```python
from build123d import *

# Parameters (mm, degrees)
CROQUIS1_R                   = 5.9
SALIENTE_EXTRUIR1_DEPTH      = 32.5
CORTAR_EXTRUIR1_DEPTH        = 24
CORTAR_EXTRUIR_L_MINA1_START = -6.5
CROQUIS3_R                   = 5.8
CROQUIS3_R_2                 = 5
CORTAR_EXTRUIR_L_MINA1_DEPTH = 3
CROQUIS4_W                   = 7
CROQUIS4_H                   = 7
SALIENTE_EXTRUIR2_DEPTH      = 7
CROQUIS6_R                   = 1.75
CORTAR_EXTRUIR3_DEPTH        = 10.4
CORTAR_EXTRUIR4_DEPTH        = 18


with BuildPart() as part:
    # Croquis1 → Saliente-Extruir1 (new body, symmetric)
    with BuildSketch(Plane.XY):
        Circle(CROQUIS1_R)
    extrude(amount=SALIENTE_EXTRUIR1_DEPTH, both=True)

    # Croquis2 → Cortar-Extruir1 (cut)
    with BuildSketch(Plane.XY):
        with BuildLine():
            Line((-5.9, 0), (5.9, 0))
            ThreePointArc((5.9, 0), (0, 5.9), (-5.9, 0))
        make_face()
    extrude(amount=-CORTAR_EXTRUIR1_DEPTH, mode=Mode.SUBTRACT)

    # Croquis3 → Cortar-Extruir-L_mina1 (cut)
    with BuildSketch(Plane.XY.offset(32.5).offset(CORTAR_EXTRUIR_L_MINA1_START)):
        Circle(CROQUIS3_R)
        Circle(CROQUIS3_R_2, mode=Mode.SUBTRACT)
    extrude(amount=-CORTAR_EXTRUIR_L_MINA1_DEPTH, mode=Mode.SUBTRACT)

    # Croquis4 → Saliente-Extruir2 (add)
    with BuildSketch(Plane.XY.offset(32.5)):
        Rectangle(CROQUIS4_W, CROQUIS4_H)
    extrude(amount=SALIENTE_EXTRUIR2_DEPTH)

    # Croquis6 → Cortar-Extruir3 (cut, through all)
    with BuildSketch(Plane.ZY.offset(3.5)):
        with Locations((36.5, 0)):
            Circle(CROQUIS6_R)
    extrude(amount=-CORTAR_EXTRUIR3_DEPTH, mode=Mode.SUBTRACT)

    # Croquis2_2 → Cortar-Extruir4 (cut)
    with BuildSketch(Plane.XY):
        with BuildLine():
            Line((-5.9, 0), (5.9, 0))
            ThreePointArc((5.9, 0), (0, 5.9), (-5.9, 0))
        make_face()
    extrude(amount=CORTAR_EXTRUIR4_DEPTH, mode=Mode.SUBTRACT)


solid = part.part
```
The listing builds one solid part. Answer for the finished solid, in the listing's coordinates (mm). A direction names the side the tool comes from. Coordinates: 2 decimals unless noted, no trailing zeros. Write each loop counter-clockwise with the first axis right and the second up, starting at its lowest first coordinate (ties: lowest second). Pieces come first, ordered by that corner, then holes. Notation, with made-up numbers: (89.25, -14.75) -> (109.25, -14.75) arc R20 cw to (109.25, 3.25) -> close; hole circle Ø3 at (-22.5, -1). An arc over 180 degrees is marked (long way). Write each question's results on one line, items separated by ' | '. Start each with the question number.
1) A cutting plane is placed at B-B (x = 0). Determine the outline of the cut face in (y, z).
2) A tool of negligible diameter and unlimited length cuts with its end or side. For faces 4 (the flat face through (2, 5, 26)), 5 (the flat face through (3.5, 0, 34)), 6 (the flat face through (0, -3.5, 36)), from which of +Z, -Z, +X, -X, +Y, -Y can it reach the whole face along a straight path? Write none if from no direction.
3) For a pull along Y with two mould halves and no side action, classify faces 1 (the cylindrical face through (-1.08, -4.88, 24.52)), 2 (the flat face through (0, 3.5, 36)), 3 (the flat face through (-3.5, 0, 34)) as +Y half, -Y half, draft (parallel to the pull), parting line (faces both ways), or undercut.
4) Flat-ended cylindrical pins translate along their axes: pin 1 Ø4 at (x, z) = (-0.5, -12.5) entering from +Y; pin 2 Ø3.5 at (y, z) = (1.5, 37) entering from +X; pin 3 Ø3 at (x, z) = (4.5, -11.5) entering from -Y. Find the tip coordinate at first contact, or state that the pin passes through.
5) A cutting plane is placed at A-A (z = 36.5). Determine the outline of the cut face in (x, y).
6) A cutting plane is placed at C-C (y = -2.5). Determine the outline of the cut face in (x, z).
7) A cutting plane is placed at D-D (z = 24.5). Determine the outline of the cut face in (x, y).
8) Straight lines are drawn through the part: probe 1 along Z at (x, y) = (-5.25, 1.75); probe 2 along Z at (x, y) = (1.25, 1.25); probe 3 along Y at (x, z) = (-1, 36.5). For each, find the intervals that lie inside material, in ascending order.
Values follow:
1) outline: (-5.9, -32.5) -> (5.9, -32.5) -> (5.9, -24) -> (0, -24) -> (0, 18) -> (5.9, 18) -> (5.9, 32.5) -> (3.5, 32.5) -> (3.5, 39.5) -> (-3.5, 39.5) -> (-3.5, 32.5) -> (-5.9, 32.5) -> close; hole (-5.8, 23) -> (-5, 23) -> (-5, 26) -> (-5.8, 26) -> close; hole circle Ø3.5 at (0, 36.5); hole (5, 23) -> (5.8, 23) -> (5.8, 26) -> (5, 26) -> close
2) face 4: none | face 5: +Z, +X, +Y, -Y | face 6: +Z, +X, -X, -Y
3) face 1: undercut | face 2: +Y half | face 3: draft
4) pin 1: y = 0 | pin 2: x = 3.5 | pin 3: y = -5.08
5) outline: (-3.5, -3.5) -> (3.5, -3.5) -> (3.5, -1.75) -> (-3.5, -1.75) -> close; (-3.5, 1.75) -> (3.5, 1.75) -> (3.5, 3.5) -> (-3.5, 3.5) -> close
6) outline: (-5.34, -32.5) -> (5.34, -32.5) -> (5.34, 32.5) -> (3.5, 32.5) -> (3.5, 39.5) -> (-3.5, 39.5) -> (-3.5, 32.5) -> (-5.34, 32.5) -> close; hole (-5.23, 23) -> (-4.33, 23) -> (-4.33, 26) -> (-5.23, 26) -> close; hole (4.33, 23) -> (5.23, 23) -> (5.23, 26) -> (4.33, 26) -> close
7) outline: circle Ø11.8 at (0, 0); circle Ø10 at (0, 0); hole circle Ø11.6 at (0, 0)
8) probe 1: -32.5 to -24, 18 to 23, 26 to 32.5 | probe 2: -32.5 to -24, 18 to 35.28, 37.72 to 39.5 | probe 3: -3.5 to -1.75, 1.75 to 3.5
